Check sheet for the drawn part. Datum: minimum x, y, z corner. Units: mm. Give positions to 0.01 mm unless a question says otherwise; leave off trailing zeros. Write each loop counter-clockwise with the first axis right and the second up, starting at its lowest first coordinate (ties: lowest second). Pieces come first, ordered by that corner, then holes. Notation, with made-up numbers: (-16.75, 9) -> (14.25, 9) arc R22 cw to (14.25, 36) -> close; hole circle Ø1 at (-24.75, 59). An arc over 180 degrees is marked (long way). Write item = value, one per line. Start each with the question number.
1. Thickness scan on line 1 along X through (y, z) = (0.5, 3.75); line 2 along X through (y, z) = (0.15, 4.5); line 3 along Z through (x, y) = (3.5, 0.5). Record the ranges inside material, lowest first.
2. Cross-section at C-C, the plane z = 4. Record the cut outline in (x, y).
3. Cross-section at D-D, the plane z = 0.5. Record the cut outline in (x, y), plus the area to 3 significant figures.
4. Cross-section at B-B, the plane y = 0.55. Record the cut outline in (x, z).
5. Cross-section at A-A, the plane x = 15. Record the cut outline in (y, z), plus the area to 3 significant figures.
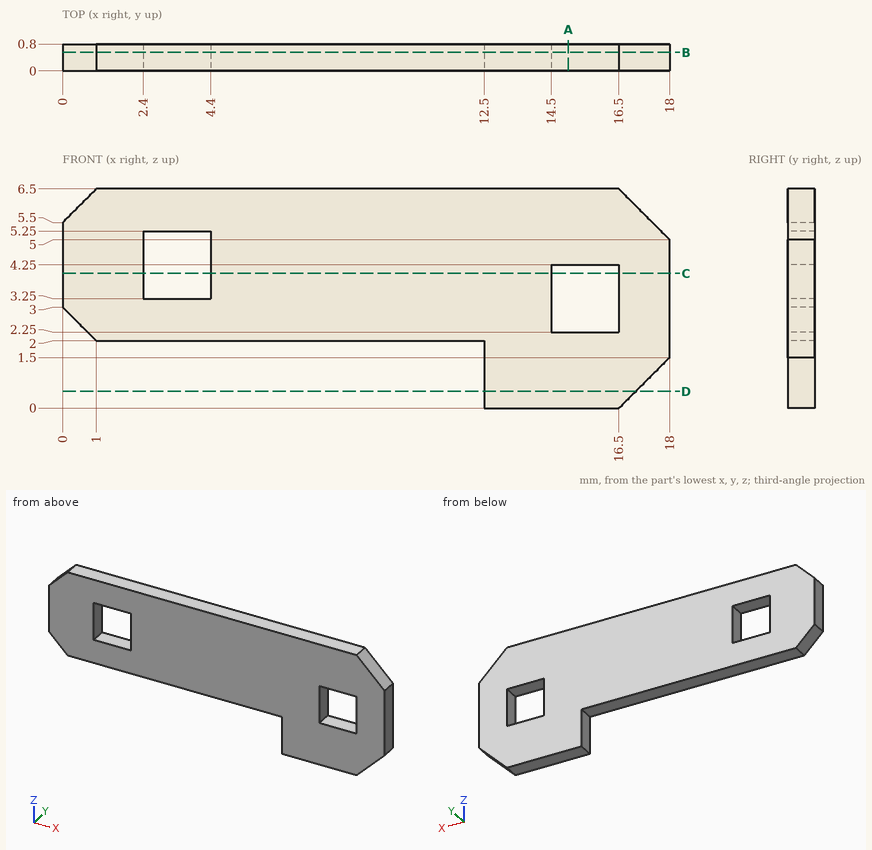
Answers:
q1.line_1 = 0 to 2.4, 4.4 to 14.5, 16.5 to 18
q1.line_2 = 0 to 2.4, 4.4 to 18
q1.line_3 = 2 to 3.25, 5.25 to 6.5
q2.outline = (0, 0) -> (2.4, 0) -> (2.4, 0.8) -> (0, 0.8) -> close; (4.4, 0) -> (14.5, 0) -> (14.5, 0.8) -> (4.4, 0.8) -> close; (16.5, 0) -> (18, 0) -> (18, 0.8) -> (16.5, 0.8) -> close
q3.outline = (12.5, 0) -> (17, 0) -> (17, 0.8) -> (12.5, 0.8) -> close
q3.area = 3.60 mm^2
q4.outline = (0, 3) -> (1, 2) -> (12.5, 2) -> (12.5, 0) -> (16.5, 0) -> (18, 1.5) -> (18, 5) -> (16.5, 6.5) -> (1, 6.5) -> (0, 5.5) -> close; hole (2.4, 3.25) -> (4.4, 3.25) -> (4.4, 5.25) -> (2.4, 5.25) -> close; hole (14.5, 2.25) -> (16.5, 2.25) -> (16.5, 4.25) -> (14.5, 4.25) -> close
q5.outline = (0, 0) -> (0.8, 0) -> (0.8, 2.25) -> (0, 2.25) -> close; (0, 4.25) -> (0.8, 4.25) -> (0.8, 6.5) -> (0, 6.5) -> close
q5.area = 3.60 mm^2
